Geometry: final body of the model. Coordinates: model frame, mm. A direction names the side the tool comes from. Give positions to 0.01 mm unless a question says otherwise; leave off trailing zeros. Order: outer loops, then holes, each group sorted by start corner. A loop starts at its lowest first (then second) coordinate and runs counter-clockwise, first axis right, second up. Notation, with made-up numbers: (20.25, 88.5) - (49.25, 88.5) arc R29 cw to (49.25, 123.5) - close; hole circle Ø3 at (-18, 22.5). An arc over 180 degrees is marked (long way). One line per question, with ' | ' between items. Start each with the question number.
Autodesk Inventor part; units mm, degrees
ref_plane "Work Plane1" through (0, 0, -6) normal (0, 0, 1) x (1, 0, 0)
ref_plane "YZ Plane" through (0, 0, 0) normal (1, 0, 0) x (0, 1, 0)
ref_plane "XZ Plane" through (0, 0, 0) normal (0, 1, 0) x (-1, 0, 0)
sketch "Sketch1" plane through (0, 0, 0) normal (0, 0, 1) x (1, 0, 0)
  circle A0 centre (0, 0) radius 7
  circle A1 centre (0, 65) radius 3
  line L0 (-57.25, -10) -> (57.25, -10)
  line L1 (57.25, -10) -> (57.25, 90)
  line L2 (57.25, 90) -> (-57.25, 90)
  line L3 (-57.25, 90) -> (-57.25, -10)
  line L4 (0, 65) -> (0, 0) construction
  point P0 (0, 32.5)
  point P1 (-57.25, 40)
  point P2 (0, 90)
  dimension "d0" = 14
  dimension "d1" = 6
  dimension "d2" = 65
  dimension "d3" = 114.5
  dimension "d7" = 25
  dimension "d8" = 10
extrude "Extrusion1" add sketch "Sketch1" along normal blind 10
sketch "Sketch2" plane through (-57.25, -10, 0) normal (0, -1, 0) x (1, 0, 0)
  line L0 (0, 10) -> (114.5, 10)
  line L1 (0, 10) -> (114.5, 10)
  line L2 (114.5, 10) -> (114.5, -35)
  line L3 (114.5, -35) -> (0, -35)
  line L4 (0, -35) -> (0, 10)
  point P0 (57.25, 0)
  point P1 (114.5, 0)
  dimension "d10" = 45
extrude "Extrusion2" add sketch "Sketch2" along normal blind 10
sketch "Sketch3" plane through (0, 0, 0) normal (0, 0, -1) x (-1, 0, 0)
  circle A0 centre (0, 0) radius 22.5 construction
  circle A1 centre (0, 0) radius 7
  line L0 (-22.5, 0) -> (-22.5, -10)
  line L1 (57.25, -10) -> (-57.25, -10) construction
  line L2 (22.5, 0) -> (22.5, -10)
  arc A2 (22.5, 0) -> (-22.5, 0) centre (0, 0) ccw
  line L3 (-22.5, -10) -> (22.5, -10)
  dimension "d13" = 45
extrude "Extrusion3" add sketch "Sketch3" along normal blind 35
sketch "Sketch4" plane through (-57.25, 90, 0) normal (-1, 0, 0) x (0, 0, 1)
  line L0 (-35, -100) -> (0, -100)
  line L1 (-35, -100) -> (0, 0)
  line L2 (0, 0) -> (10, 0)
  line L3 (0, 0) -> (10, 0)
  line L4 (10, 0) -> (10, -110)
  line L5 (10, 0) -> (10, -110)
  line L6 (10, -110) -> (-35, -110)
  line L7 (10, -110) -> (-35, -110)
  line L8 (-35, -100) -> (-35, -110)
  line L9 (-35, -110) -> (-35, -100)
extrude "Extrusion4" add sketch "Sketch4" against normal blind 10
sketch "Sketch5" plane through (57.25, 90, 10) normal (1, 0, 0) x (0, 0, -1)
  line L0 (45, -100) -> (10, 0)
  line L1 (10, -100) -> (10, 0)
  line L2 (45, -100) -> (10, -100)
  point P0 (0, -110)
extrude "Extrusion5" add sketch "Sketch5" against normal blind 10
sketch "Sketch9" plane through (0, 0, 0) normal (0, 0, -1) x (-1, 0, 0)
  circle A0 centre (0, 72) radius 20
  circle A1 centre (0, 65) radius 3
  point P0 (0, 0)
  dimension "d28" = 40
  dimension "d95" = 7
extrude "Extrusion8" cut sketch "Sketch9" against normal blind 1 contours A0 | A1
sketch "Sketch10" plane through (-57.25, -10, 0) normal (0, 1, 0) x (1, 0, 0)
  circle A0 centre (83.5, 20) radius 2
  line L0 (0, 0) -> (0, 35)
  circle A1 centre (31, 20) radius 2
  line L1 (34.75, 35) -> (79.75, 35)
  line L2 (34.75, 35) -> (79.75, 35)
  line L3 (83.5, 20) -> (31, 20)
  line L4 (79.75, 35) -> (34.75, 35)
  point P0 (57.25, 0)
  point P1 (114.5, 35)
  point P2 (57.25, 20)
  point P3 (57.25, 35)
  dimension "d31" = 4
  dimension "d33" = 4
  dimension "d55" = 15
  dimension "d57" = 52.5
extrude "Extrusion9" cut sketch "Sketch10" against normal through all
sketch "Sketch11" plane through (0, 0, -35) normal (0, 0, -1) x (-1, 0, 0)
  line L0 (57.25, -20) -> (-57.25, -20)
  line L1 (-57.25, -20) -> (-57.25, -39)
  line L2 (-57.25, -39) -> (57.25, -39)
  line L3 (57.25, -39) -> (57.25, -20)
  point P0 (0, 0)
  point P1 (57.25, -20)
  point P2 (-57.25, -20)
  point P3 (0, -20)
  dimension "d36" = 19
extrude "Extrusion10" add sketch "Sketch11" against normal blind 8.5
sketch "Sketch12" plane through (0, 0, -35) normal (0, 0, -1) x (-1, 0, 0)
  circle A0 centre (-35, -29) radius 2
  circle A1 centre (35, -29) radius 2
  line L0 (-35, -29) -> (35, -29) construction
  line L1 (-57.25, -39) -> (57.25, -39)
  point P0 (0, 0)
  point P1 (0, -29)
  point P2 (0, -39)
  dimension "d39" = 4
  dimension "d40" = 4
  dimension "d41" = 70
  dimension "d42" = 10
extrude "Extrusion11" cut sketch "Sketch12" against normal through all
ref_plane "Work Plane1" through (0, 0, -6) normal (0, 0, 1) x (1, 0, 0)
sketch "Sketch14" plane through (0, 0, -6) normal (0, 0, 1) x (1, 0, 0)
  circle A0 centre (35, -29) radius 2
  circle A1 centre (-35, -29) radius 2
  line L0 (-57.25, -20) -> (57.25, -20)
  line L1 (-57.25, -20) -> (-57.25, -39)
  line L2 (-57.25, -39) -> (57.25, -39)
  line L3 (57.25, -39) -> (57.25, -20)
  point P0 (0, 0)
extrude "Extrusion12" add sketch "Sketch14" along normal blind 10 contours A0 | A1 | L0 L3 L2 L1
sketch "Sketch15" plane through (0, 0, 4) normal (0, 0, 1) x (1, 0, 0)
  circle A0 centre (0, -29) radius 2
  line L0 (-57.25, -39) -> (57.25, -39)
  point P0 (0, 0)
  point P1 (0, -39)
  dimension "d48" = 4
  dimension "d49" = 10
extrude "Extrusion13" cut sketch "Sketch15" against normal blind 10
sketch "Sketch16" plane through (0, 0, 4) normal (0, 0, 1) x (1, 0, 0)
  circle A0 centre (0, -29) radius 2
  line L0 (-57.25, -20) -> (57.25, -20)
  line L1 (-57.25, -20) -> (-57.25, -39)
  line L2 (-57.25, -39) -> (57.25, -39)
  line L3 (57.25, -39) -> (57.25, -20)
  circle A1 centre (0, -29) radius 2
  circle A2 centre (0, -29) radius 7.5
  point P0 (0, 0)
  dimension "d52" = 15
extrude "Extrusion14" add sketch "Sketch16" along normal blind 6 contours L0 L3 L2 L1
sketch "Sketch17" plane through (-57.25, -10, 0) normal (0, 1, 0) x (1, 0, 0)
  line L0 (114.5, 6) -> (0, 6)
  line L1 (0, 6) -> (0, 26.5)
  line L2 (0, 26.5) -> (114.5, 26.5)
  line L3 (114.5, 26.5) -> (114.5, 6)
  circle A0 centre (83.5, 20) radius 2
  circle A1 centre (31, 20) radius 2
  line L4 (0, 6) -> (0, 26.5)
  line L5 (0, 26.5) -> (-36.5, -10) construction
  line L6 (0, 26.5) -> (51.6188, 26.5) construction
  line L7 (114.5, -10) -> (0, -10)
  line L8 (0, -10) -> (-36.5, -10) construction
  line L9 (0, 26.5) -> (0, -10)
  line L10 (114.5, 26.5) -> (114.5, 6)
  line L11 (114.5, 26.5) -> (151, -10) construction
  line L12 (114.5, -10) -> (151, -10) construction
  line L13 (114.5, -10) -> (114.5, 26.5)
  line L14 (129.5, 11.5) -> (129.5, -10)
  line L15 (114.5, 26.5) -> (129.5, 11.5)
  line L16 (129.5, -10) -> (114.5, -10)
  line L17 (-15, 11.5) -> (-15, -10)
  line L18 (0, 35) -> (0, 26.5)
  line L19 (0, 26.5) -> (-15, 11.5)
  line L20 (0, -10) -> (-15, -10)
  point P0 (57.25, 0)
  dimension "d58" = 135
  dimension "d60" = 135
  dimension "d65" = 15
  dimension "d66" = 15
extrude "Extrusion15" add sketch "Sketch17" along normal blind 100 contours L3 L15 L14 L16 L13 | L9 L20 L17 L19 L1
sketch "Sketch18" plane through (57.25, 14.2857, -26.5) normal (-1, 0, 0) x (0, 0, 1)
  line L0 (26.5, 75.7143) -> (-8.5, -24.2857) construction
  line L1 (26.5, -24.2857) -> (-8.5, -24.2857) construction
  line L2 (26.5, 75.7143) -> (26.5, -24.2857) construction
  line L3 (-8.5, -24.2857) -> (-8.5, 75.7143)
  line L4 (-8.5, 75.7143) -> (26.5, 75.7143)
  line L5 (-8.5, -24.2857) -> (26.5, 75.7143)
extrude "Extrusion16" cut sketch "Sketch18" along normal through all both and the other way through all
sketch "Sketch19" plane through (-72.25, -10, -11.5) normal (-0.7071, 0, -0.7071) x (-0.7071, 0, 0.7071)
  circle A0 centre (-10.6066, 15) radius 1.5
  line L0 (-21.2132, 0) -> (0, 0)
  point P0 (-42.9567, 10)
  point P1 (-10.6066, 0)
  dimension "d67" = 3
  dimension "d68" = 15
extrude "Extrusion17" cut sketch "Sketch19" against normal through all
sketch "Sketch20" plane through (72.25, -10, -11.5) normal (0.7071, 0, -0.7071) x (-0.7071, 0, -0.7071)
  circle A0 centre (10.6066, 15) radius 1.5
  line L0 (0, 0) -> (21.2132, 0)
  point P0 (42.9567, 10)
  point P1 (10.6066, 0)
  dimension "d71" = 3
  dimension "d72" = 15
extrude "Extrusion18" cut sketch "Sketch20" against normal through all
sketch "Sketch21" plane through (-47.25, 90, 0) normal (0, 1, 0) x (1, 0, 0)
  line L0 (-25, -10) -> (-10, -10)
  line L1 (-25, -10) -> (-19.6967, -4.6967) construction
  line L2 (-25, -10) -> (-17.5, -10) construction
  line L3 (-25, 11.5) -> (-25, -10)
  line L4 (-25, 0.6066) -> (-14.3934, -10)
  line L5 (-25, 0.6066) -> (-25, -10)
  line L6 (-14.3934, -10) -> (-25, -10)
  line L7 (-25, -10) -> (119.5, -10)
  line L8 (119.5, -10) -> (114.1967, -4.6967) construction
  line L9 (119.5, -10) -> (127, -10) construction
  line L10 (108.8934, -10) -> (119.5, 0.6066)
  line L11 (119.5, -10) -> (119.5, 11.5)
  line L12 (108.8934, -10) -> (123.8934, -10) construction
  line L13 (108.8934, -10) -> (119.5, -10)
  line L14 (119.5, -10) -> (119.5, 0.6066)
  point P0 (47.25, 0)
  dimension "d75" = 7.5
  dimension "d76" = 45
  dimension "d77" = 7.5
  dimension "d78" = 135
  dimension "d79" = 45
extrude "Extrusion19" cut sketch "Sketch21" against normal through all
sketch "Sketch22" plane through (0, 0, 10) normal (0, 0, 1) x (1, 0, 0)
  circle A0 centre (0, 0) radius 14.5
  circle A1 centre (0, 0) radius 7
  dimension "d82" = 29
extrude "Extrusion20" cut sketch "Sketch22" against normal blind 8
sketch "Sketch23" plane through (-47.25, -10, -35) normal (0, 0, -1) x (-1, 0, 0)
  circle A0 centre (-47.25, 10) radius 7
  circle A1 centre (-47.25, 10) radius 14.5
  dimension "d85" = 29
extrude "Extrusion21" cut sketch "Sketch23" against normal blind 16.5
sketch "Sketch24" plane through (0, 72, 1) normal (0, 0, -1) x (-1, 0, 0)
  circle A0 centre (0, -7) radius 3
  circle A1 centre (0, -7) radius 6.5
  point P0 (0, -72)
  dimension "d88" = 13
extrude "Extrusion22" cut sketch "Sketch24" against normal blind 7
sketch "Sketch27" plane through (0, 0, 1) normal (0, 0, -1) x (-1, 0, 0)
  arc A0 (-8.7178, 90) -> (8.7178, 90) centre (0, 72) ccw construction
  circle A1 centre (15.5, 72) radius 2
  circle A2 centre (7.75, 85.4234) radius 2
  circle A3 centre (-7.75, 85.4234) radius 2
  circle A4 centre (-15.5, 72) radius 2
  circle A5 centre (-7.75, 58.5766) radius 2
  circle A6 centre (7.75, 58.5766) radius 2
  point P0 (0, 0)
  dimension "d96" = 4
  dimension "d97" = 15.5
  dimension "d100" = 360
extrude "Extrusion24" cut sketch "Sketch27" against normal blind 10
sketch "Sketch28" plane through (0, 0, 10) normal (0, 0, 1) x (1, 0, 0)
  circle A0 centre (-7.75, 85.4234) radius 2
  circle A1 centre (7.75, 85.4234) radius 2
  circle A2 centre (15.5, 72) radius 2
  circle A3 centre (7.75, 58.5766) radius 2
  circle A4 centre (-7.75, 58.5766) radius 2
  circle A5 centre (-15.5, 72) radius 2
  circle A6 centre (15.5, 72) radius 3.5
  arc A7 (-8.7178, 90) -> (8.7178, 90) centre (0, 72) ccw construction
  circle A8 centre (7.75, 85.4234) radius 3.5
  circle A9 centre (-7.75, 85.4234) radius 3.5
  circle A10 centre (-15.5, 72) radius 3.5
  circle A11 centre (-7.75, 58.5766) radius 3.5
  circle A12 centre (7.75, 58.5766) radius 3.5
  point P0 (0, 0)
  dimension "d104" = 7
  dimension "d107" = 360
extrude "Extrusion25" cut sketch "Sketch28" against normal blind 3 contours A0 | A1 | A2 | A3 | A4 | A5 | A6 | A8 | A9 | A10 | A11 | A12
properties part number "WA004" material "ABS Plastic"
(1) Cut plane C-C, the plane y = 37. Return the cut outline in (x, z).
(2) Pull-direction query (Y, two-part tool) for faces 5 (the cylindrical face through (18.733, 70.659, 8.521)), 6 (the cylindrical face through (0.495, 22.495, -12.03)), 7 (the flat face through (-57.25, -18, -13)), 8 (the cylindrical face through (34.077, -30.774, -30.81)); classes: +Y half, -Y half, draft (parallel to the pull), parting line (faces both ways), or undercut.
(3) Access query for faces 1 (the flat face through (-1, -31, -6)), 2 (the cylindrical face through (-35.923, -30.774, -30.81)), 3 (the flat face through (35, -10, -17)), 4 (the cylindrical face through (7.294, 62.047, 8.521)). Directions: +Z, -Z, +X, -X, +Y, -Y. A direction counts if a zero-diameter tool reaches every point of the face in a straight line with its end or side. Return the directions, or none.
(4) Material intervals for line 1 along X through (y, z) = (-15, -20); line 2 along X through (y, z) = (8, -8.5); line 3 along X through (y, z) = (34, -1.5), sorted ascending. Write a range as from..to.
(5) Contact query for flat-ended pins moving along their axis: P1, Ø5, axis at x = -7.75, y = 85.42, coming from the +Z side; P2, Ø3.5, axis at x = -7.75, y = 58.58, coming from the -Z side; P3, Ø1, axis at x = 37, y = 69, coming from the -Z side; P4, Ø8, axis at x = 0, y = 65, coming from the -Z side. Output: stop coordinate, or through.
(6) Cut plane A-A, the plane y = -29. Return the cut outline in (x, z), plus the area to 3 significant figures.
(7) Cut plane D-D, the plane z = -15.5. Give the number of separate pieces and of enclosed holes in the cut face, plus the area to 3 significant figures.
(8) Cut plane B-B, the plane x = -26.25. Return the cut outline in (y, z).
Results are:
1) outline: (-72.25, -11.5) - (-65.2, -18.55) - (-47.25, -18.55) - (-47.25, 0) - (47.25, 0) - (47.25, -18.55) - (65.2, -18.55) - (72.25, -11.5) - (72.25, -0.61) - (61.64, 10) - (-61.64, 10) - (-72.25, -0.61) - close
2) face 5: undercut | face 6: +Y half | face 7: draft | face 8: undercut
3) face 1: +X, -X, -Y | face 2: -Z | face 3: -Z, +Y | face 4: +Z
4) line 1: -57.25..-28.25, -24.25..24.25, 28.25..57.25 | line 2: -72.25..-47.25, -21.03..21.03, 47.25..72.25 | line 3: -72.25..-47.25, 47.25..72.25
5) P1: z = 7 | P2: through | P3: z = 0 | P4: z = 8
6) outline: (-57.25, -35) - (-37, -35) - (-37, -26.5) - (-57.25, -26.5) - close; (-57.25, -6) - (-2, -6) - (-2, 4) - (-7.5, 4) - (-7.5, 10) - (-57.25, 10) - close; (-33, -35) - (33, -35) - (33, -26.5) - (-33, -26.5) - close; (2, -6) - (57.25, -6) - (57.25, 10) - (7.5, 10) - (7.5, 4) - (2, 4) - close; (37, -35) - (57.25, -35) - (57.25, -26.5) - (37, -26.5) - close | area: 2,610 mm2
7) separate pieces: 1 | enclosed holes: 3 | area: 4,560 mm2
8) outline: (-39, -35) - (-10, -35) - (-10, -22) - (-20, -22) - (-20, -26.5) - (-39, -26.5) - close; (-39, -6) - (-20, -6) - (-20, -18) - (-10, -18) - (-10, 0) - (90, 0) - (90, 10) - (-39, 10) - close
